Can you work these out from the drawing? Everything is in mm from the part's minimum corner. A direction names the side the tool comes from. Give positions to 0.01 mm unless a question says otherwise; leave off trailing zeros. Order: outer loops, then holes, each group sorted by start corner. A loop starts at its lowest first (then second) coordinate and runs counter-clockwise, first axis right, second up. Notation, with made-up numbers: M 35,-5 L 49,-5 A19 ccw 49,7 Z; hole C 85,-17 d7. An arc over 180 degrees is marked long. Answer as a JSON object with one key per item and string values.
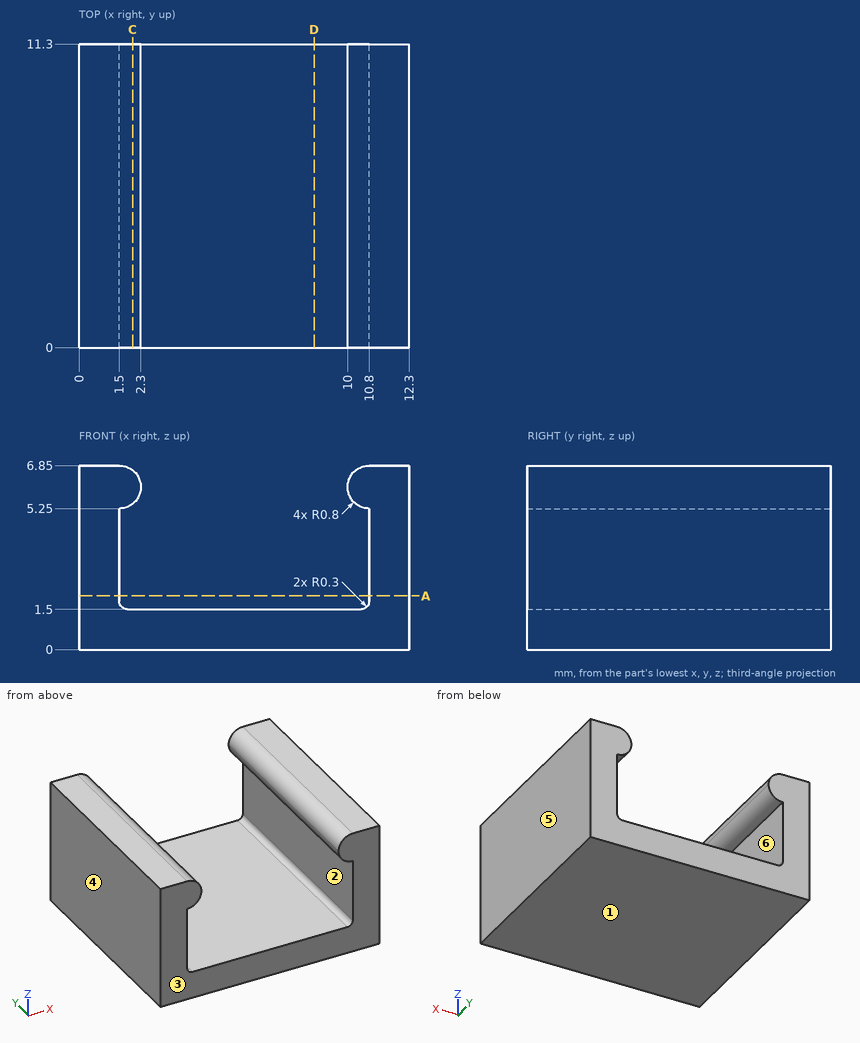
1) Thinking about a two-plate mould opening in X: for the marked faces 3, 4, 5 and 6, which applies, pulls with the +X half, pulls with the -X half, needs draft (parallel to the pull), parting line crosses it, or undercut?
Results found:
{"face 3": "needs draft", "face 4": "pulls with the -X half", "face 5": "pulls with the +X half", "face 6": "undercut"}
2) I'm going to push flat-ended pins straight in: pin 1 Ø2 at (x, z) = (5, 5) entering from -Y; pin 2 Ø3 at (x, y) = (4, 4.5) entering from +Z. Where does each tip first touch, or does it pass through?
Results found:
{"pin 1": "passes through", "pin 2": "stops at z = 1.5"}
3) I want a section at C-C on x = 2. Write out the boundary of the cut face in (y, z), and give its area (3 significant figures).
Results found:
{"outline": "M 0,0 L 11.3,0 L 11.3,1.5 L 0,1.5 Z; M 0,5.43 L 11.3,5.43 L 11.3,6.67 L 0,6.67 Z", "area": "31.1 mm²"}
4) I want a section at D-D on x = 8.75. Write out the boundary of the cut face in (y, z).
Results found:
{"outline": "M 0,0 L 11.3,0 L 11.3,1.5 L 0,1.5 Z"}
5) I want a section at A-A on z = 2. Write out the boundary of the cut face in (x, y), and give its area (3 significant figures).
Results found:
{"outline": "M 0,0 L 1.5,0 L 1.5,11.3 L 0,11.3 Z; M 10.8,0 L 12.3,0 L 12.3,11.3 L 10.8,11.3 Z", "area": "33.9 mm²"}
6) For the marked faces 1 and 2, which set-ups out of +Z, -Z, +X, -X, +Y, -Y let a thin tool reach every point of the face, with its end or its side?
Results found:
{"face 1": "-Z, +X, -X, +Y, -Y", "face 2": "+Y, -Y"}
7) I need wall thicknesses on L1, parallel to X at y = 4, z = 3.5; L2, parallel to Z at x = 7.75, y = 10.75; L3, parallel to X at y = 4.25, z = 6. Which ranges of each line are inside material? Lowest first, please.
Results found:
{"L1": "x = 0 to 1.5, 10.8 to 12.3", "L2": "z = 0 to 1.5", "L3": "x = 0 to 2.3, 10 to 12.3"}
